```python
from build123d import *

# Parameters (mm, degrees)
CYLINDER001_R     = 3
CYLINDER001_DEPTH = 1
CYLINDER004_R     = 3
CYLINDER004_DEPTH = 3
CYLINDER003_R     = 3
CYLINDER003_DEPTH = 3
CYLINDER002_R     = 7
CYLINDER002_DEPTH = 3
CHAMFER_SIZE      = 1


with BuildPart() as cilindro001:
    # Cylinder001 → Cylinder001 (new body)
    with BuildSketch(Plane(origin=(4, 16, -1), x_dir=(1, 0, 0), z_dir=(0, 0, 1))):
        Circle(CYLINDER001_R)
    extrude(amount=CYLINDER001_DEPTH)


with BuildPart() as cilindro004:
    # Cylinder004 → Cylinder004 (new body)
    with BuildSketch(Plane(origin=(4, 9, -3), x_dir=(1, 0, 0), z_dir=(0, 0, 1))):
        Circle(CYLINDER004_R)
    extrude(amount=CYLINDER004_DEPTH)


with BuildPart() as cilindro003:
    # Cylinder003 → Cylinder003 (new body)
    with BuildSketch(Plane(origin=(4, 23, -3), x_dir=(1, 0, 0), z_dir=(0, 0, 1))):
        Circle(CYLINDER003_R)
    extrude(amount=CYLINDER003_DEPTH)


with BuildPart() as chamfer_body:
    # Cylinder002 → Cylinder002 (new body)
    with BuildSketch(Plane(origin=(4, 16, -3), x_dir=(1, 0, 0), z_dir=(0, 0, 1))):
        Circle(CYLINDER002_R)
    extrude(amount=CYLINDER002_DEPTH)

    # Cut003: cut Cilindro003
    add(cilindro003.part, mode=Mode.SUBTRACT)

    # Cut004: cut Cilindro004
    add(cilindro004.part, mode=Mode.SUBTRACT)

    # Cut005: cut Cilindro001
    add(cilindro001.part, mode=Mode.SUBTRACT)

    # Chamfer
    chamfer_edges = [chamfer_body.edges().sort_by_distance(p)[0] for p in [
        (6.930313, 22.357143, -1.5),
        (1.069687, 22.357143, -1.5),
        (6.930313, 9.642857, -1.5),
        (1.069687, 9.642857, -1.5),
    ]]
    chamfer(chamfer_edges, length=CHAMFER_SIZE)


with BuildPart() as chamfer_body_1:
    # Chamfer placement: moved
    add(chamfer_body.part.moved(Location((-38, 1, 3))))


solid = chamfer_body_1.part
```
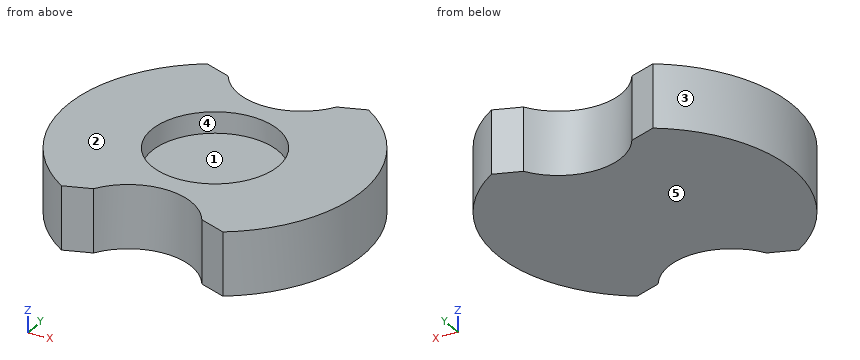
Geometry: final body of the model. Coordinates: model frame, mm. Face numbers are marked on the shaded views. A direction names the side the tool comes from. Coordinates: 2 decimals unless noted, no trailing zeros. Order: outer loops, then holes, each group sorted by start corner. A loop starts at its lowest first (then second) coordinate and runs counter-clockwise, first axis right, second up. Notation, with made-up numbers: (45, 23) -> (81, 23) arc R34 ccw to (81, 62) -> close; hole circle Ø9 at (35.25, 31). An arc over 180 degrees is marked (long way). Write each question's results on one line, items separated by ' | '. Start each with the question number.
1) Mould query, pull axis X, two halves, no side actions, for the marked faces 3, 4 and 5. Classes: released by +X, released by -X, zero draft, split by the parting line, or undercut.
2) Cut plane C-C, the plane x = -30. Output: boundary loops of the cut face in (y, z).
3) Cut plane D-D, the plane y = 13.75. Output: boundary loops of the cut face in (x, z).
4) First-contact query: pin 1 (1.5 mm diameter, centred on x = -31, y = 17.5, fed in from -Z); pin 2 (1 mm diameter, centred on x = -39.5, z = 1, fed in from -Y); pin 3 (1.8 mm diameter, centred on x = -32.5, y = 17.5, fed in from +Z). Flat tips, straight axial feed; report the tip coordinate or a pass-through.
5) Material intervals for line 1 along Z through (x, y) = (-34.5, 17); line 2 along Y through (x, z) = (-33.25, 2.3); line 3 along X through (y, z) = (17.5, 2.65), sorted ascending.
6) Cut plane A-A, the plane x = -34. Output: boundary loops of the cut face in (y, z), and give its area (3 significant figures).
7) Set-up query: the marked faces 1 and 2. Return all of +Z, -Z, +X, -X, +Y, -Y with unobstructed straight access to the full face (end or side cutting, diameter ignored); none if empty.
8) Cut plane B-B, the plane y = 17. Output: boundary loops of the cut face in (x, z), and give its area (3 significant figures).
Checks:
1) face 3: released by -X | face 4: undercut | face 5: zero draft
2) outline: (11.26, 0) -> (22.74, 0) -> (22.74, 3) -> (11.26, 3) -> close
3) outline: (-40.2, 0) -> (-27.8, 0) -> (-27.8, 3) -> (-40.2, 3) -> close
4) pin 1: z = 0 | pin 2: y = 12.1 | pin 3: z = 2
5) line 1: 0 to 2 | line 2: 12.9 to 14.1, 19.9 to 21.1 | line 3: -40.98 to -36.96, -31.04 to -27.02
6) outline: (13, 0) -> (21, 0) -> (21, 3) -> (20, 3) -> (20, 2) -> (14, 2) -> (14, 3) -> (13, 3) -> close | area: 18.0 mm^2
7) face 1: +Z | face 2: +Z, +X, -X, +Y, -Y
8) outline: (-41, 0) -> (-27, 0) -> (-27, 3) -> (-31, 3) -> (-31, 2) -> (-37, 2) -> (-37, 3) -> (-41, 3) -> close | area: 36.0 mm^2
